The listing builds one solid part. Answer for the finished solid, in the listing's coordinates (mm). A direction names the side the tool comes from. Round coordinates to 2 decimals unless told otherwise and drop trailing zeros. Write each loop counter-clockwise with the first axis right and the second up, starting at its lowest first coordinate (ties: lowest second). Pieces come first, ordered by that corner, then holes.
Item 1: A tool of negligible diameter and unlimited length cuts with its end or side. For faces 1 (the face through (-4, 0, 4)), 2 (the face through (4.632, -0.173, 0.135)), from which of +Z, -Z, +X, -X, +Y, -Y can it reach the whole face along a straight path? Write none if from no direction.
Item 2: Find the intervals of material crossed by probe 1 along Y at (x, z) = (-4, 105.5); probe 2 along Y at (x, z) = (-3.75, 80.5), in increasing order.
Item 3: Find section A-A on z = 28. Give the vertices of the cut face in (x, y), then the cut area to 3 significant figures.
Item 4: Each of these flat-tipped pins is pushed along its axis until it touches: pin 1 (1 mm diameter, centred on y = -2, z = 91.5, fed in from +X); pin 2 (2 mm diameter, centred on x = 3.5, z = 98, fed in from -Y); pin 3 (1 mm diameter, centred on x = 2, z = 96, fed in from -Y). Where does it stop, or does it pass through?
```python
from build123d import *

# Parameters (mm, degrees)
SKETCH1_R           = 5
BOSS_EXTRUDE1_DEPTH = 145
CUT_EXTRUDE1_DEPTH  = 8
CHAMFER1_SIZE       = 0.5


with BuildPart() as part:
    # Sketch1 → Boss-Extrude1 (new body)
    with BuildSketch(Plane.XY):
        Circle(SKETCH1_R)
    extrude(amount=BOSS_EXTRUDE1_DEPTH)

    # Sketch2 → Cut-Extrude1 (cut)
    with BuildSketch(Plane(origin=(0, 0, 0), x_dir=(-1, 0, 0), z_dir=(0, 0, -1))):
        with BuildLine():
            Line((4, 3), (4, -3))
            ThreePointArc((4, -3), (5, 0), (4, 3))
        make_face()
    extrude(amount=-CUT_EXTRUDE1_DEPTH, mode=Mode.SUBTRACT)

    # Chamfer1
    chamfer1_edges = [part.edges().sort_by_distance(p)[0] for p in [
        (-5, 0, 145),
        (1.58113883, 4.74341649, 0),
    ]]
    chamfer(chamfer1_edges, length=CHAMFER1_SIZE)


solid = part.part
```
Check values:
1. face 1: -Z, -X, +Y, -Y
1. face 2: -Z
2. probe 1: y = -3 to 3
2. probe 2: y = -3.31 to 3.31
3. outline: circle Ø10 at (0, 0)
3. area: 78.5 mm2
4. pin 1: stops at x = 4.77
4. pin 2: stops at y = -4.33
4. pin 3: stops at y = -4.77
